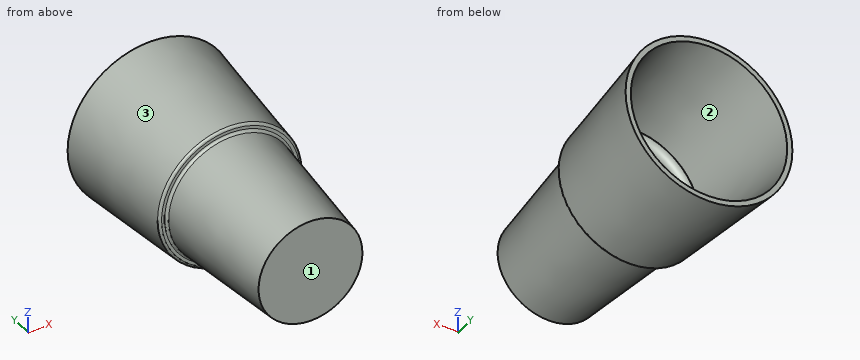
```python
from build123d import *

# Parameters (mm, degrees)
FILLET1_R = 1.27
SHELL1_T  = -2.54


with BuildPart() as part:
    # Sketch1 → Revolve2 (revolve)
    with BuildSketch(Plane.XY, mode=Mode.PRIVATE) as revolve2_sk:
        Polygon((0, 0), (25.4, 0), (31.185877256, 63.5), (34.995877256, 63.5), (40.781754513, 127), (0, 127), align=None)
    revolve(revolve2_sk.sketch.rotate(Axis((0, 0, 0), (0, 1, 0)), 90), axis=Axis((0, 0, 0), (0, 1, 0)))

    # Fillet1
    fillet1_edges = [part.edges().sort_by_distance(p)[0] for p in [
        (0, 63.5, 34.995877256),
        (0, 63.5, 31.185877256),
    ]]
    fillet(fillet1_edges, radius=FILLET1_R)

    # Shell1
    shell1_openings = [part.faces().sort_by_distance(p)[0] for p in [
        (0, 127, 0),
    ]]
    offset(amount=SHELL1_T, openings=shell1_openings, kind=Kind.INTERSECTION)


solid = part.part
```
Can you work these out from the model? Positions are in its coordinate system, mm. Face numbers are marked on the shaded views. Round coordinates to 2 decimals unless told otherwise and drop trailing zeros. Loops run counter-clockwise (first coordinate to the right, second up) from the corner with the lowest first, then second, coordinate; pieces in that order, holes last. Notation, with made-up numbers: (52.25, 80.5) -> (109.25, 80.5) arc R18 cw to (109.25, 113.5) -> close; hole circle Ø8 at (-8.75, 58). An arc over 180 degrees is marked (long way). One line per item, written item: value. Start each with the question number.
1. If we section it at B-B, the plane x = 0: Write out the boundary of the cut face in (y, z).
2. For pin 1 (8 mm diameter, centred on x = 24.5, y = 69, fed in from +Z); pin 2 (5 mm diameter, centred on y = 18, z = 2, fed in from +X); pin 3 (1.5 mm diameter, centred on y = 111.5, z = -1.5, fed in from +X), each with a flat end and sliding along its axis, tell me the tip position at first contact or that it passes through.
3. If I drill on probe 1 along Z at (x, y) = (-15.5, 64.5); probe 2 along Z at (x, y) = (2, 27); probe 3 along X at (y, z) = (102, -25), over which ranges is the centre line in solid material (lowest first)?
4. If we mould it in two halves opening along X, with no side actions, what happens to the marked faces 1, 2 and 3? For each: pulls with the +X half, pulls with the -X half, needs draft (parallel to the pull), parting line crosses it, or undercut.
5. If we section it at D-D, the plane y = 80: Write out the boundary of the cut face in (x, z), then the cut area to 3 significant figures.
6. If we section it at C-C, the plane y = 24: Write out the boundary of the cut face in (x, z).
7. If we section it at A-A, the plane z = 0: Write out the boundary of the cut face in (x, y).
Calculated:
1. outline: (0, -25.4) -> (62.35, -31.08) arc R1.27 cw to (63.5, -32.35) -> (63.5, -33.84) arc R1.27 ccw to (64.65, -35.1) -> (127, -40.78) -> (127, -38.23) -> (66.04, -32.68) -> (66.04, -32.35) arc R3.81 ccw to (62.58, -28.55) -> (2.54, -23.08) -> (2.54, 23.08) -> (62.58, 28.55) arc R3.81 ccw to (66.04, 32.35) -> (66.04, 32.68) -> (127, 38.23) -> (127, 40.78) -> (64.65, 35.1) arc R1.27 ccw to (63.5, 33.84) -> (63.5, 32.35) arc R1.27 cw to (62.35, 31.08) -> (0, 25.4) -> close
2. pin 1: stops at z = 29.01
2. pin 2: stops at x = 27.23
2. pin 3: stops at x = 39.41
3. probe 1: z = -31.47 to -24.85, 24.85 to 31.47
3. probe 2: z = -27.79 to -25.23, 25.23 to 27.79
3. probe 3: x = -29.28 to -25.84, 25.84 to 29.28
4. face 1: needs draft
4. face 2: undercut
4. face 3: parting line crosses it
5. outline: circle Ø73 at (0, 0); hole circle Ø67.9 at (0, 0)
5. area: 564 mm²
6. outline: circle Ø55.17 at (0, 0); hole circle Ø50.07 at (0, 0)
7. outline: (-40.78, 127) -> (-35.1, 64.65) arc R1.27 ccw to (-33.84, 63.5) -> (-32.35, 63.5) arc R1.27 cw to (-31.08, 62.35) -> (-25.4, 0) -> (25.4, 0) -> (31.08, 62.35) arc R1.27 cw to (32.35, 63.5) -> (33.84, 63.5) arc R1.27 ccw to (35.1, 64.65) -> (40.78, 127) -> (38.23, 127) -> (32.68, 66.04) -> (32.35, 66.04) arc R3.81 ccw to (28.55, 62.58) -> (23.08, 2.54) -> (-23.08, 2.54) -> (-28.55, 62.58) arc R3.81 ccw to (-32.35, 66.04) -> (-32.68, 66.04) -> (-38.23, 127) -> close
